```python
from build123d import *

# Parameters (mm, degrees)
SKETCH1_W             = 17.78
SKETCH1_H             = 50.8
SKETCH1_R             = 2.032
BOSS_EXTRUDE1_DEPTH   = 3.96875
SKETCH3_W             = 17.78
SKETCH3_H             = 25.4
SKETCH2_W             = 17.78
SKETCH2_H             = 29.21
SKETCH4_W             = 13.716
SKETCH4_H             = 2.032
BOSS_EXTRUDE2_DEPTH   = 2.54
EXTRUDE_THIN1_DEPTH   = 14.2875
FILLET1_R             = 2.54
CUT_EXTRUDE1_DEPTH    = 0.9525
SKETCH8_R             = 1.27
CUT_EXTRUDE2_DEPTH    = 0.9525
BODY_MOVE_COPY3_ANGLE = 90


with BuildPart() as part:
    # Sketch1 → Boss-Extrude1 (new body)
    with BuildSketch(Plane.XY):
        Rectangle(SKETCH1_W, SKETCH1_H)
        with Locations((0, 18.796)):
            Circle(SKETCH1_R, mode=Mode.SUBTRACT)
        with Locations((0, -18.796)):
            Circle(SKETCH1_R, mode=Mode.SUBTRACT)
    extrude(amount=BOSS_EXTRUDE1_DEPTH)

    # Sketch3 → Loft1 section 0
    with BuildSketch(Plane.XY.offset(10.795)):
        Rectangle(SKETCH3_W, SKETCH3_H)
    # Sketch2 → Loft1 section 1
    with BuildSketch(Plane.XY.offset(3.96875)):
        Rectangle(SKETCH2_W, SKETCH2_H)
    loft()

    # Sketch4 → Boss-Extrude2 (add)
    with BuildSketch(Plane.XY.offset(10.795)):
        with Locations((0, 9.271)):
            Rectangle(SKETCH4_W, SKETCH4_H)
        with Locations((0, -9.271)):
            Rectangle(SKETCH4_W, SKETCH4_H)
    extrude(amount=BOSS_EXTRUDE2_DEPTH)


with BuildPart() as body_2:
    # Sketch6 → Extrude-Thin1 (new body, symmetric)
    with BuildSketch(Plane(origin=(0, 0, 0), x_dir=(1, 0, 0), z_dir=(0, 1, 0))):
        with BuildLine():
            Line((9.525, -13.335), (-6.985, -13.335))
            ThreePointArc((-6.985, -13.335), (-8.781051224, -14.078948776), (-9.525, -15.875))
            Line((-9.525, -15.875), (-9.525, -31.877))
            Line((-9.525, -31.877), (-8.5725, -31.877))
            Line((-8.5725, -31.877), (-8.5725, -15.875))
            ThreePointArc((-8.5725, -15.875), (-8.107532015, -14.752467985), (-6.985, -14.2875))
            Line((-6.985, -14.2875), (9.525, -14.2875))
            Line((9.525, -14.2875), (9.525, -13.335))
        make_face()
    extrude(amount=EXTRUDE_THIN1_DEPTH, both=True)

    # Fillet1
    fillet1_edges = [body_2.edges().sort_by_distance(p)[0] for p in [
        (9.525, 14.2875, 13.81125),
        (-9.04875, 14.2875, 31.877),
        (9.525, -14.2875, 13.81125),
        (-9.04875, -14.2875, 31.877),
    ]]
    fillet(fillet1_edges, radius=FILLET1_R)

    # Sketch7 → Cut-Extrude1 (cut)
    with BuildSketch(Plane.ZY.offset(9.525)):
        with BuildLine():
            Line((19.304, 11.303), (25.273, 11.303))
            ThreePointArc((25.273, 11.303), (27.051, 9.525), (25.273, 7.747))
            Line((25.273, 7.747), (19.304, 7.747))
            ThreePointArc((19.304, 7.747), (17.526, 9.525), (19.304, 11.303))
        make_face()
        with BuildLine():
            Line((19.304, -7.747), (25.273, -7.747))
            ThreePointArc((25.273, -7.747), (27.051, -9.525), (25.273, -11.303))
            Line((25.273, -11.303), (19.304, -11.303))
            ThreePointArc((19.304, -11.303), (17.526, -9.525), (19.304, -7.747))
        make_face()
    extrude(amount=-CUT_EXTRUDE1_DEPTH, mode=Mode.SUBTRACT)

    # Sketch8 → Cut-Extrude2 (cut)
    with BuildSketch(Plane(origin=(-8.5725, 0, 0), x_dir=(0, 0, -1), z_dir=(1, 0, 0))):
        with Locations((-29.083, 0)):
            Circle(SKETCH8_R)
    extrude(amount=-CUT_EXTRUDE2_DEPTH, mode=Mode.SUBTRACT)


with BuildPart() as body_2_1:
    # Body-Move/Copy1: moved
    add(body_2.part.moved(Location((0, 0, 25.4))))


with BuildPart() as part_1:
    # Body-Move/Copy3: moved
    add(part.part.rotate(Axis((0, 0, 0), (0, 0, 1)), BODY_MOVE_COPY3_ANGLE))


solid = part_1.part
```
Input: part model. Units: mm. Frame: model coordinates. A direction names the side the tool comes from. Give positions to 0.01 mm unless a question says otherwise; leave off trailing zeros. Order: outer loops, then holes, each group sorted by start corner. A loop starts at its lowest first (then second) coordinate and runs counter-clockwise, first axis right, second up. Notation, with made-up numbers: (9, 66) - (58, 66) arc R15 ccw to (58, 72) - close; hole circle Ø3 at (-19, 2). An arc over 180 degrees is marked (long way). Use a Markdown table: item, result.
(1) Access query for faces 4 (the flat face through (-9, -6.858, 12)), 5 (the flat face through (9, 6.858, 12)), 6 (the flat face through (10.287, 0, 12)), 7 (the flat face through (-10.287, 0, 12)). Directions: +Z, -Z, +X, -X, +Y, -Y. A direction counts if a zero-diameter tool reaches every point of the face in a straight line with its end or side. Return the directions, or none.
Computed values:
| item | result |
|---|---|
| face 4 | +Z, +X, -X, -Y |
| face 5 | +Z, +X, -X, +Y |
| face 6 | +Z, +X, +Y, -Y |
| face 7 | +Z, -X, +Y, -Y |
(2) Section query C-C (y = 4.25). Output: boundary loops of the cut face in (x, z) (3 decimals), then the cut area to 3 significant figures.
Computed values:
| item | result |
|---|---|
| outline | (-25.4, 0) - (25.4, 0) - (25.4, 3.969) - (14.605, 3.969) - (12.7, 10.795) - (10.287, 10.795) - (10.287, 13.335) - (8.255, 13.335) - (8.255, 10.795) - (-8.255, 10.795) - (-8.255, 13.335) - (-10.287, 13.335) - (-10.287, 10.795) - (-12.7, 10.795) - (-14.605, 3.969) - (-25.4, 3.969) - close |
| area | 398 mm2 |
(3) Section query A-A (y = 0). Output: boundary loops of the cut face in (x, z) (3 decimals).
Computed values:
| item | result |
|---|---|
| outline | (-25.4, 0) - (-20.828, 0) - (-20.828, 3.969) - (-25.4, 3.969) - close; (-16.764, 0) - (16.764, 0) - (16.764, 3.969) - (14.605, 3.969) - (12.7, 10.795) - (10.287, 10.795) - (10.287, 13.335) - (8.255, 13.335) - (8.255, 10.795) - (-8.255, 10.795) - (-8.255, 13.335) - (-10.287, 13.335) - (-10.287, 10.795) - (-12.7, 10.795) - (-14.605, 3.969) - (-16.764, 3.969) - close; (20.828, 0) - (25.4, 0) - (25.4, 3.969) - (20.828, 3.969) - close |
(4) Line query: line 1 (X direction, y = 0, z = 1); line 2 (X direction, y = -1.25, z = 2.5); line 3 (Z direction, x = -11.5, y = -5.5) (3 decimals). Output: solid intervals per line, ascending. Write a range as from..to.
Computed values:
| item | result |
|---|---|
| line 1 | x = -25.4..-20.83, -16.76..16.76, 20.83..25.4 |
| line 2 | x = -25.4..-20.4, -17.19..17.19, 20.4..25.4 |
| line 3 | z = 0..10.795 |
(5) Pin query (flat end, axial travel): pin 1 (5.5 mm diameter, centred on x = -18.796, y = 0, fed in from -Z); pin 2 (2 mm diameter, centred on y = -0.5, z = 11.5, fed in from -X); pin 3 (3 mm diameter, centred on y = 2, z = 12.5, fed in from -X); pin 4 (5 mm diameter, centred on x = -3, y = -4.5, fed in from +Z) (3 decimals). Return the tip coordinate at first contact, or that it passes through.
Computed values:
| item | result |
|---|---|
| pin 1 | stops at z = 0 |
| pin 2 | stops at x = -12.78 |
| pin 3 | stops at x = -10.29 |
| pin 4 | stops at z = 10.795 |
(6) Draft query along X for faces 1 (the cylindrical face through (16.78, -0.26, 1.96)), 2 (the flat face through (-9, 6.858, 12)), 3 (the flat face through (-13.666, 0.124, 7.334)). Return one class per face: released by +X, released by -X, zero draft, split by the parting line, or undercut.
Computed values:
| item | result |
|---|---|
| face 1 | undercut |
| face 2 | zero draft |
| face 3 | released by -X |
(7) Section query D-D (z = 1.5). Output: boundary loops of the cut face in (x, y).
Computed values:
| item | result |
|---|---|
| outline | (-25.4, -8.89) - (25.4, -8.89) - (25.4, 8.89) - (-25.4, 8.89) - close; hole circle Ø4.06 at (-18.8, 0); hole circle Ø4.06 at (18.8, 0) |
(8) Section query B-B (z = 11.75). Output: boundary loops of the cut face in (x, y) (3 decimals).
Computed values:
| item | result |
|---|---|
| outline | (-10.287, -6.858) - (-8.255, -6.858) - (-8.255, 6.858) - (-10.287, 6.858) - close; (8.255, -6.858) - (10.287, -6.858) - (10.287, 6.858) - (8.255, 6.858) - close |
